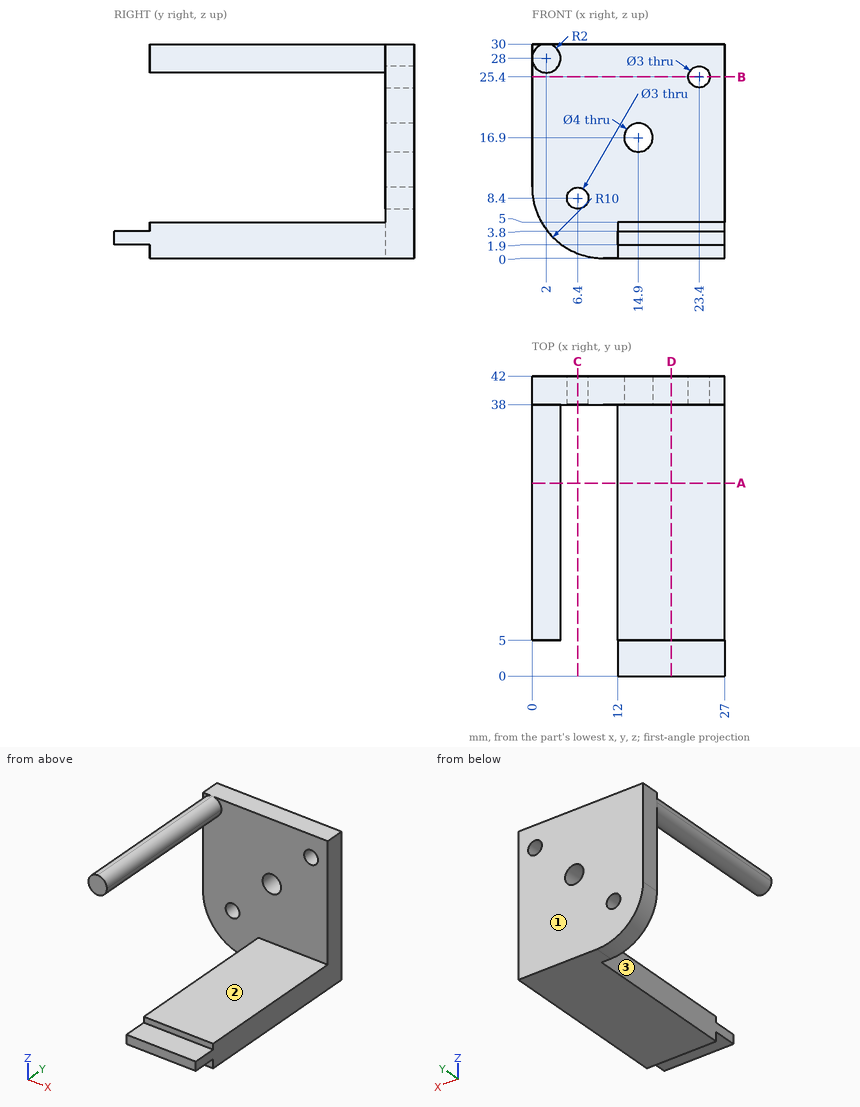
Drawing for the job (mm, zero at the part's lowest x, y, z). A direction names the side the tool comes from. Give positions to 0.01 mm unless a question says otherwise; leave off trailing zeros. Order: outer loops, then holes, each group sorted by start corner. A loop starts at its lowest first (then second) coordinate and runs counter-clockwise, first axis right, second up. Notation, with made-up numbers: (-30, -20.75) -> (21, -20.75) arc R34 cw to (21, 17.25) -> close; hole circle Ø4 at (5, 43.5). An arc over 180 degrees is marked (long way). Use one line per item in the form item = value.
(1) Saw through at B-B (z = 25.4). Write the cut outline in (x, y).
Solution:
outline = (0, 38) -> (21.9, 38) -> (21.9, 42) -> (0, 42) -> close; (24.9, 38) -> (27, 38) -> (27, 42) -> (24.9, 42) -> close
(2) Tool access for the marked faces 1, 2 and 3: list every direction of +Z, -Z, +X, -X, +Y, -Y with a clear straight run to the whole face (end or side of a thin tool).
Solution:
face_1 = +Z, -Z, +X, -X, +Y
face_2 = +Z, +X, -X, -Y
face_3 = +Z, -Z, -X, -Y
(3) Flat gauge pins, fed straight in: P1, Ø2, axis at x = 2.5, z = 28.5, coming from the -Y side; P2, Ø4.5, axis at x = 18.5, y = 16, coming from the +Z side; P3, Ø2.5, axis at x = 19, y = 3, coming from the -Z side. Where does each tip first touch, or does it go through?
Solution:
P1 = 5
P2 = 5
P3 = 1.9
(4) Saw through at D-D (x = 19.5). Write the cut outline in (y, z).
Solution:
outline = (0, 1.9) -> (5, 1.9) -> (5, 0) -> (42, 0) -> (42, 30) -> (38, 30) -> (38, 5) -> (5, 5) -> (5, 3.8) -> (0, 3.8) -> close
(5) Drill centre lines: line 1 (X direction, y = 39.5, z = 25.4); line 2 (Y direction, x = 9.5, z = 16.5); line 3 (Z direction, x = 14.25, y = 28). Where is each one in solid material? Low to high. Write a range as from..to.
Solution:
line_1 = 0..21.9, 24.9..27
line_2 = 38..42
line_3 = 0..5
(6) Saw through at A-A (y = 27). Write the cut outline in (x, z), then the cut area to 3 significant figures.
Solution:
outline = circle Ø4 at (2, 28); (12, 0) -> (27, 0) -> (27, 5) -> (12, 5) -> close
area = 87.6 mm²
(7) Saw through at C-C (x = 6.4). Write the cut outline in (y, z).
Solution:
outline = (38, 0.67) -> (42, 0.67) -> (42, 6.9) -> (38, 6.9) -> close; (38, 9.9) -> (42, 9.9) -> (42, 30) -> (38, 30) -> close
